Verification items for the finished model (mm, model axes). Face numbers are marked on the shaded views. A direction names the side the tool comes from. Round coordinates to 2 decimals unless told otherwise and drop trailing zeros. Loops run counter-clockwise (first coordinate to the right, second up) from the corner with the lowest first, then second, coordinate; pieces in that order, holes last. Notation, with made-up numbers: M 7,5 L 26,5 A17 cw 26,22 Z; hole C 87.5,86 d3. An arc over 180 degrees is marked long. One line per item, written item: value.
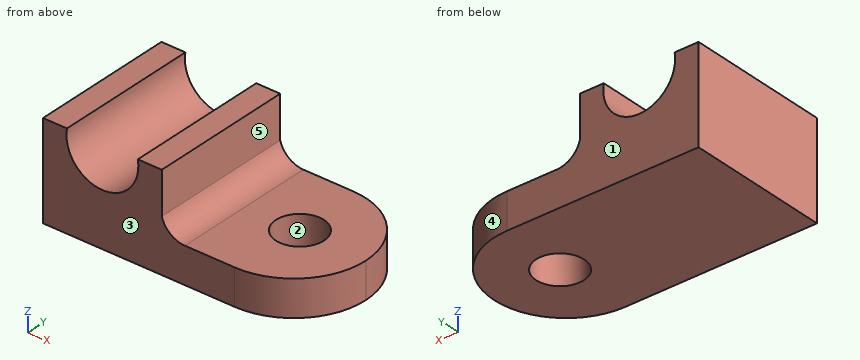
from build123d import *

# Parameters (mm, degrees)
F1_DEPTH = 76.2
F2_R     = 38.09999
F3_R     = 12.7
F4_DEPTH = 50.8
F5_DEPTH = 25.4


# Not quite as in the source:
# - a fillet or chamfer is up to 0.001 mm smaller than in the source, because OpenCascade refuses the exact size


with BuildPart() as f1:
    # F0 (on Front) → F1 (new body)
    with BuildSketch(Plane.XZ):
        with BuildLine():
            Line((-50.2547219646, 33.020831282), (-62.9547219646, 33.020831282))
            Line((-62.9547219646, 33.020831282), (-62.9547219646, -17.779168718))
            Line((-62.9547219646, -17.779168718), (76.7452780354, -17.779168718))
            Line((76.7452780354, -17.779168718), (76.7452780354, 1.270831282))
            Line((76.7452780354, 1.270831282), (12.2243361415, 1.270831282))
            ThreePointArc((12.2243361415, 1.270831282), (4.5574789786, 3.8461435711), (0, 10.5276342357))
            Line((0, 10.5276342357), (0, 33.020831282))
            Line((0, 33.020831282), (-12.7, 33.020831282))
            ThreePointArc((-12.7, 33.020831282), (-31.4773609823, 10.7594118855), (-50.2547219646, 33.020831282))
        make_face()
    extrude(amount=F1_DEPTH)

    # F2 (radius 38.1 in the source; OpenCascade refuses exactly that, so slightly less here)
    f2_edges = [f1.edges().sort_by_distance(p)[0] for p in [
        (76.745278, -76.2, -8.254169),
        (76.745278, 0, -8.254169),
    ]]
    fillet(f2_edges, radius=F2_R)

    # F3 (on Top) → F4 (cut)
    with BuildSketch(Plane.XY):
        with Locations((40.9884415567, -37.0847843587)):
            Circle(F3_R)
    extrude(amount=F4_DEPTH, mode=Mode.SUBTRACT)

    # F5 (cut): a face of the model
    f5_faces = [f1.faces().sort_by_distance(p)[0] for p in [
        (40.9884415567, -37.0847843587, 0),
    ]]
    extrude(f5_faces, amount=-F5_DEPTH, mode=Mode.SUBTRACT)


solid = f1.part
(1) Tool access check on the marked faces 4 and 5. Record the directions out of +Z, -Z, +X, -X, +Y, -Y that give a thin tool (end or side, any length) a straight path to the whole face; none if there is none.
Completed:
face 4: +Z, -Z, +X, +Y
face 5: +Z, +X, +Y, -Y
(2) Sectioned sample at C-C on z = 26. Enter the section's corners in (x, y).
Completed:
outline: M -62.95,-76.2 L -50.14,-76.2 L -50.14,0 L -62.95,0 Z; M -12.81,-76.2 L 0,-76.2 L 0,0 L -12.81,0 Z
(3) Thickness scan on L1, parallel to Z at x = 46, y = -22.5; L2, parallel to X at y = -22, z = 15.5; L3, parallel to X at y = -62.5, z = 28. Record the ranges inside material, lowest first. Write a range as from..to.
Completed:
L1: z = -17.78..1.27
L2: x = -62.95..-44.05, -18.9..0
L3: x = -62.95..-50.44, -12.51..0
(4) Sectioned sample at A-A on y = -35. Enter the section's corners in (x, z), and give its area (3 significant figures).
Completed:
outline: M -62.95,-17.78 L 28.46,-17.78 L 28.46,1.27 L 12.22,1.27 A12.7 cw 0,10.53 L 0,33.02 L -12.7,33.02 A19.05 cw long -50.25,33.02 L -62.95,33.02 Z; M 53.52,-17.78 L 76.62,-17.78 L 76.62,1.27 L 53.52,1.27 Z
area: 3,520 mm^2
(5) Sectioned sample at D-D on y = -9. Enter the section's corners in (x, z).
Completed:
outline: M -62.95,-17.78 L 63.24,-17.78 L 63.24,1.27 L 12.22,1.27 A12.7 cw 0,10.53 L 0,33.02 L -12.7,33.02 A19.05 cw long -50.25,33.02 L -62.95,33.02 Z
(6) Depth check by flat-ended pin: pin 1 Ø10 at (x, z) = (-16.5, 10) entering from +Y; pin 2 Ø23 at (x, y) = (40.99, -37.08) entering from -Z; pin 3 Ø18 at (y, z) = (-34.5, 18) entering from +X. Enter the tip coordinate at first touch or a pass-through.
Completed:
pin 1: stops at y = 0
pin 2: passes through
pin 3: stops at x = 0.54
(7) Sectioned sample at B-B on x = 33. Enter the section's corners in (y, z).
Completed:
outline: M -76.2,-17.78 L -46.96,-17.78 L -46.96,1.27 L -76.2,1.27 Z; M -27.21,-17.78 L 0,-17.78 L 0,1.27 L -27.21,1.27 Z
(8) Mould release check, pull along Y, two halves, no side actions. Record for the marked faces 1, 2 and 3: +Y half, -Y half, draft (parallel to the pull), parting line (faces both ways), or undercut.
Completed:
face 1: +Y half
face 2: undercut
face 3: -Y half
